For this review, take the finished solid that the model builds, in its own axes (mm). Face numbers are marked on the shaded views. A direction names the side the tool comes from. Round coordinates to 2 decimals unless told otherwise and drop trailing zeros. Write each loop counter-clockwise with the first axis right and the second up, starting at its lowest first coordinate (ties: lowest second). Pieces come first, ordered by that corner, then holes. Notation, with made-up numbers: M -20.75,-40 L -5.75,-40 A21 ccw -5.75,-4 Z; hole C 54,27 d7. An arc over 180 degrees is marked long. Use one line per item in the form item = value. Start each with the question number.
Item 1: Draft analysis for pull direction Y (two halves, no side actions). For the marked faces 6, 7, 8 and 9, state which applies: released by +Y, released by -Y, zero draft, split by the parting line, or undercut.
Item 2: Add section C-C (y = -3694). State the section outline as (x, z) points.
Item 3: For P1, Ø5, axis at x = 7373, y = -3677.5, coming from the +Z side; P2, Ø3.5, axis at x = 7512, z = 29, coming from the -Y side; P3, Ø24, axis at x = 7526.5, y = -3762, coming from the +Z side; P4, Ø3.5, axis at x = 7403.5, z = 28, coming from the -Y side, all flat-tipped, find the tip position at first contact; note any pin that passes through.
Item 4: For line 1 (Y direction, x = 7536.5, z = 31); line 2 (X direction, y = -3691, z = 32.5); line 3 (Y direction, x = 7405, z = 28), list the stretches that pass through material, from the lowest coordinate up. Write a range as [from, to].
Item 5: Add section A-A (z = 97.5). State the section outline as (x, y) points, and give its area (3 significant figures).
Item 6: For the marked faces 1, 2, 3, 4 and 5, list the 3-axis set-ups (+Z, -Z, +X, -X, +Y, -Y) from which the entire face can be reached by the end or side of a thin tool; tool diameter is ignored.
Item 7: Add section B-B (x = 7409). State the section outline as (y, z) points, and give its area (3 significant figures).
Item 8: Add section D-D (z = 14). State the section outline as (x, y) points, and give its area (3 significant figures).
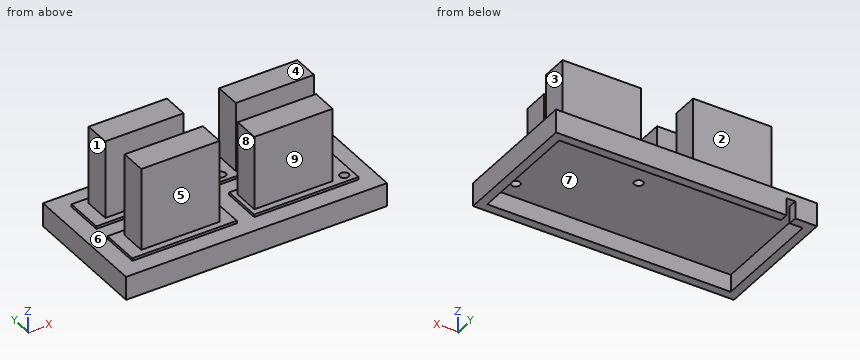
Autodesk Inventor part; units mm, degrees
ref_plane "YZ Plane" through (0, 0, 0) normal (1, 0, 0) x (0, 1, 0)
ref_plane "XZ Plane" through (0, 0, 0) normal (0, 1, 0) x (-1, 0, 0)
ref_plane "XY Plane" through (0, 0, 0) normal (0, 0, 1) x (1, 0, 0)
sketch "Skizze1" plane through (0, 0, 0) normal (0, 0, 1) x (1, 0, 0)
  line L0 (7309.0058, -3653.1811) -> (7609.0058, -3653.1811)
  line L1 (7609.0058, -3653.1811) -> (7609.0058, -3803.1811)
  line L2 (7609.0058, -3803.1811) -> (7309.0058, -3803.1811)
  line L3 (7309.0058, -3803.1811) -> (7309.0058, -3653.1811)
  point P0 (0, 0)
  dimension "d0" = 300
  dimension "d1" = 150
extrude "Extrusion1" add sketch "Skizze1" along normal blind 30
sketch "Skizze2" plane through (0, 0, 30) normal (0, 0, 1) x (1, 0, 0)
  line L0 (7309.0058, -3653.1811) -> (7309.0058, -3803.1811)
  line L1 (7609.0058, -3803.1811) -> (7609.0058, -3653.1811)
  line L2 (7309.0058, -3718.1811) -> (7609.0058, -3718.1811)
  line L3 (7609.0058, -3718.1811) -> (7609.0058, -3738.1811)
  line L4 (7609.0058, -3738.1811) -> (7309.0058, -3738.1811)
  line L5 (7309.0058, -3738.1811) -> (7309.0058, -3718.1811)
  line L6 (7609.0058, -3653.1811) -> (7309.0058, -3653.1811)
  point P0 (0, 0)
  dimension "d4" = 20
  dimension "d5" = 65
extrude "Extrusion2" cut sketch "Skizze2" against normal blind 3 contours L2 L1 L4 L0
sketch "Skizze3" plane through (0, 0, 30) normal (0, 0, 1) x (1, 0, 0)
  line L0 (7609.0058, -3653.1811) -> (7309.0058, -3653.1811)
  line L1 (7309.0058, -3803.1811) -> (7609.0058, -3803.1811)
  line L2 (7449.0058, -3653.1811) -> (7469.0058, -3653.1811)
  line L3 (7469.0058, -3653.1811) -> (7469.0058, -3803.1811)
  line L4 (7469.0058, -3803.1811) -> (7449.0058, -3803.1811)
  line L5 (7449.0058, -3803.1811) -> (7449.0058, -3653.1811)
  line L6 (7309.0058, -3653.1811) -> (7309.0058, -3718.1811)
  point P0 (0, 0)
  dimension "d8" = 20
  dimension "d9" = 140
extrude "Extrusion3" cut sketch "Skizze3" against normal blind 3
sketch "Skizze4" plane through (0, 0, 30) normal (0, 0, 1) x (1, 0, 0)
  line L0 (7609.0058, -3653.1811) -> (7309.0058, -3653.1811)
  line L1 (7309.0058, -3803.1811) -> (7609.0058, -3803.1811)
  line L2 (7609.0058, -3653.1811) -> (7589.0058, -3653.1811)
  line L3 (7589.0058, -3653.1811) -> (7589.0058, -3803.1811)
  line L4 (7589.0058, -3803.1811) -> (7609.0058, -3803.1811)
  line L5 (7609.0058, -3803.1811) -> (7609.0058, -3653.1811)
  line L6 (7309.0058, -3653.1811) -> (7329.0058, -3653.1811)
  line L7 (7329.0058, -3653.1811) -> (7329.0058, -3803.1811)
  line L8 (7329.0058, -3803.1811) -> (7309.0058, -3803.1811)
  line L9 (7309.0058, -3803.1811) -> (7309.0058, -3653.1811)
  line L10 (7309.0058, -3803.1811) -> (7609.0058, -3803.1811)
  line L11 (7609.0058, -3803.1811) -> (7609.0058, -3783.1811)
  line L12 (7609.0058, -3783.1811) -> (7309.0058, -3783.1811)
  line L13 (7309.0058, -3783.1811) -> (7309.0058, -3803.1811)
  line L14 (7609.0058, -3653.1811) -> (7309.0058, -3653.1811)
  line L15 (7309.0058, -3653.1811) -> (7309.0058, -3673.1811)
  line L16 (7309.0058, -3673.1811) -> (7609.0058, -3673.1811)
  line L17 (7609.0058, -3673.1811) -> (7609.0058, -3653.1811)
  point P0 (0, 0)
  point P1 (7589.0058, -3783.1811)
  point P2 (7329.0058, -3783.1811)
  point P3 (7329.0058, -3673.1811)
  point P4 (7589.0058, -3673.1811)
  dimension "d12" = 20
  dimension "d13" = 20
  dimension "d14" = 20
  dimension "d15" = 20
extrude "Extrusion4" cut sketch "Skizze4" against normal blind 3 contours L5 L16 L3 L0 | L3 L16 L7 L0 | L5 L12 L3 L16 | L7 L16 L9 L0 | L5 L1 L3 L12 | L7 L12 L9 L16 | L3 L1 L7 L12 | L7 L1 L9 L12
sketch "Skizze5" plane through (0, 0, 30) normal (0, 0, 1) x (1, 0, 0)
  line L0 (7344.0058, -3680.6811) -> (7434.0058, -3680.6811)
  line L1 (7434.0058, -3680.6811) -> (7434.0058, -3710.6811)
  line L2 (7434.0058, -3710.6811) -> (7344.0058, -3710.6811)
  line L3 (7344.0058, -3710.6811) -> (7344.0058, -3680.6811)
  line L4 (7449.0058, -3673.1811) -> (7329.0058, -3673.1811)
  line L5 (7329.0058, -3673.1811) -> (7329.0058, -3718.1811)
  line L6 (7344.0058, -3745.6811) -> (7434.0058, -3745.6811)
  line L7 (7434.0058, -3745.6811) -> (7434.0058, -3775.6811)
  line L8 (7434.0058, -3775.6811) -> (7344.0058, -3775.6811)
  line L9 (7344.0058, -3775.6811) -> (7344.0058, -3745.6811)
  line L10 (7449.0058, -3738.1811) -> (7329.0058, -3738.1811)
  line L11 (7449.0058, -3783.1811) -> (7449.0058, -3738.1811)
  line L12 (7474.0058, -3745.6811) -> (7564.0058, -3745.6811)
  line L13 (7564.0058, -3745.6811) -> (7564.0058, -3775.6811)
  line L14 (7564.0058, -3775.6811) -> (7474.0058, -3775.6811)
  line L15 (7474.0058, -3775.6811) -> (7474.0058, -3745.6811)
  line L16 (7589.0058, -3738.1811) -> (7469.0058, -3738.1811)
  line L17 (7469.0058, -3738.1811) -> (7469.0058, -3783.1811)
  line L18 (7494.0058, -3680.6811) -> (7584.0058, -3680.6811)
  line L19 (7584.0058, -3680.6811) -> (7584.0058, -3710.6811)
  line L20 (7584.0058, -3710.6811) -> (7494.0058, -3710.6811)
  line L21 (7494.0058, -3710.6811) -> (7494.0058, -3680.6811)
  line L22 (7589.0058, -3673.1811) -> (7469.0058, -3673.1811)
  line L23 (7589.0058, -3718.1811) -> (7589.0058, -3673.1811)
  line L24 (7609.0058, -3803.1811) -> (7309.0058, -3803.1811)
  line L25 (7309.0058, -3803.1811) -> (7309.0058, -3653.1811)
  line L26 (7609.0058, -3653.1811) -> (7609.0058, -3803.1811)
  line L27 (7309.0058, -3653.1811) -> (7609.0058, -3653.1811)
  point P0 (0, 0)
  point P1 (7329.0058, -3695.6811)
  point P2 (7564.0058, -3760.6811)
  dimension "d18" = 90
  dimension "d19" = 30
  dimension "d20" = 7.5
  dimension "d21" = 15
  dimension "d22" = 90
  dimension "d23" = 30
  dimension "d24" = 7.5
  dimension "d25" = 15
  dimension "d26" = 90
  dimension "d27" = 30
  dimension "d28" = 7.5
  dimension "d29" = 5
  dimension "d30" = 90
  dimension "d31" = 30
  dimension "d32" = 7.5
  dimension "d33" = 5
  dimension "d58" = 27.5
  dimension "d59" = 35
  dimension "d60" = 35
  dimension "d61" = 45
  dimension "d62" = 27.5
  dimension "d63" = 25
  dimension "d64" = 27.5
extrude "Extrusion5" add sketch "Skizze5" along normal blind 90 contours L0 L1 L2 L3
extrude "Extrusion6" add sketch "Skizze5" along normal blind 80 contours L18 L19 L20 L21
extrude "Extrusion7" add sketch "Skizze5" along normal blind 95 contours L6 L7 L8 L9
extrude "Extrusion8" add sketch "Skizze5" along normal blind 85 contours L12 L13 L14 L15
sketch "Skizze6" plane through (0, 0, 0) normal (0, 0, -1) x (-1, 0, 0)
  line L0 (-7599.0058, -3663.1811) -> (-7319.0058, -3663.1811)
  line L1 (-7319.0058, -3663.1811) -> (-7319.0058, -3793.1811)
  line L2 (-7319.0058, -3793.1811) -> (-7599.0058, -3793.1811)
  line L3 (-7599.0058, -3793.1811) -> (-7599.0058, -3663.1811)
  line L4 (-7609.0058, -3653.1811) -> (-7309.0058, -3653.1811)
  line L5 (-7609.0058, -3803.1811) -> (-7609.0058, -3653.1811)
  line L6 (-7344.0058, -3653.1811) -> (-7334.0058, -3653.1811)
  line L7 (-7334.0058, -3653.1811) -> (-7334.0058, -3663.1811)
  line L8 (-7334.0058, -3663.1811) -> (-7344.0058, -3663.1811)
  line L9 (-7344.0058, -3663.1811) -> (-7344.0058, -3653.1811)
  line L10 (-7309.0058, -3653.1811) -> (-7309.0058, -3803.1811)
  point P0 (0, 0)
  point P1 (-7334.0058, -3658.1811)
  dimension "d42" = 280
  dimension "d43" = 130
  dimension "d44" = 10
  dimension "d45" = 10
  dimension "d46" = 10
  dimension "d47" = 25
extrude "Extrusion9" cut sketch "Skizze6" against normal blind 20
sketch "Skizze7" plane through (0, 0, 30) normal (0, 0, 1) x (1, 0, 0)
  circle A0 centre (7479.0058, -3708.1811) radius 5
  circle A1 centre (7579.0058, -3773.1811) radius 5
  line L0 (7469.0058, -3673.1811) -> (7469.0058, -3718.1811)
  line L1 (7469.0058, -3718.1811) -> (7589.0058, -3718.1811)
  line L2 (7589.0058, -3783.1811) -> (7589.0058, -3738.1811)
  line L3 (7469.0058, -3783.1811) -> (7589.0058, -3783.1811)
  point P0 (0, 0)
  dimension "d50" = 10
  dimension "d51" = 10
  dimension "d52" = 10
  dimension "d53" = 10
  dimension "d54" = 10
  dimension "d55" = 10
extrude "Extrusion10" cut sketch "Skizze7" against normal through all
sketch "Skizze8" plane through (0, 0, 20) normal (0, 0, -1) x (-1, 0, 0)
  line L0 (-7349.0058, -3685.6811) -> (-7429.0058, -3685.6811)
  line L1 (-7429.0058, -3685.6811) -> (-7429.0058, -3705.6811)
  line L2 (-7429.0058, -3705.6811) -> (-7349.0058, -3705.6811)
  line L3 (-7349.0058, -3705.6811) -> (-7349.0058, -3685.6811)
  line L4 (-7609.0058, -3653.1811) -> (-7344.0058, -3653.1811)
  line L5 (-7309.0058, -3653.1811) -> (-7309.0058, -3803.1811)
  line L6 (-7349.0058, -3770.6811) -> (-7429.0058, -3770.6811)
  line L7 (-7429.0058, -3770.6811) -> (-7429.0058, -3750.6811)
  line L8 (-7429.0058, -3750.6811) -> (-7349.0058, -3750.6811)
  line L9 (-7349.0058, -3750.6811) -> (-7349.0058, -3770.6811)
  line L10 (-7309.0058, -3803.1811) -> (-7609.0058, -3803.1811)
  line L11 (-7559.0058, -3770.6811) -> (-7479.0058, -3770.6811)
  line L12 (-7479.0058, -3770.6811) -> (-7479.0058, -3750.6811)
  line L13 (-7479.0058, -3750.6811) -> (-7559.0058, -3750.6811)
  line L14 (-7559.0058, -3750.6811) -> (-7559.0058, -3770.6811)
  line L15 (-7609.0058, -3803.1811) -> (-7609.0058, -3653.1811)
  line L16 (-7499.0058, -3705.6811) -> (-7579.0058, -3705.6811)
  line L17 (-7579.0058, -3705.6811) -> (-7579.0058, -3685.6811)
  line L18 (-7579.0058, -3685.6811) -> (-7499.0058, -3685.6811)
  line L19 (-7499.0058, -3685.6811) -> (-7499.0058, -3705.6811)
  point P0 (0, 0)
  dimension "d65" = 80
  dimension "d66" = 20
  dimension "d67" = 32.5
  dimension "d68" = 40
  dimension "d69" = 80
  dimension "d70" = 20
  dimension "d71" = 40
  dimension "d72" = 32.5
  dimension "d73" = 80
  dimension "d74" = 50
  dimension "d75" = 32.5
  dimension "d76" = 80
  dimension "d77" = 20
  dimension "d78" = 32.5
  dimension "d79" = 30
extrude "Extrusion11" add sketch "Skizze8" against normal blind 70
properties part number "2"
Calculated:
q1.face_6 = undercut
q1.face_7 = undercut
q1.face_8 = zero draft
q1.face_9 = released by -Y
q2.outline = M 7309.01,0 L 7319.01,0 L 7319.01,20 L 7599.01,20 L 7599.01,0 L 7609.01,0 L 7609.01,27 L 7589.01,27 L 7589.01,30 L 7584.01,30 L 7584.01,110 L 7494.01,110 L 7494.01,30 L 7469.01,30 L 7469.01,27 L 7449.01,27 L 7449.01,30 L 7434.01,30 L 7434.01,120 L 7344.01,120 L 7344.01,30 L 7329.01,30 L 7329.01,27 L 7309.01,27 Z
q3.P1 = 30
q3.P2 = -3783.18
q3.P3 = 115
q3.P4 = -3803.18
q4.line_1 = [-3775.68, -3745.68], [-3710.68, -3680.68]
q4.line_2 = [7344.01, 7434.01], [7494.01, 7584.01]
q4.line_3 = [-3783.18, -3738.18], [-3718.18, -3673.18]
q5.outline = M 7344.01,-3775.68 L 7434.01,-3775.68 L 7434.01,-3745.68 L 7344.01,-3745.68 Z; M 7344.01,-3710.68 L 7434.01,-3710.68 L 7434.01,-3680.68 L 7344.01,-3680.68 Z; M 7474.01,-3775.68 L 7564.01,-3775.68 L 7564.01,-3745.68 L 7474.01,-3745.68 Z; M 7494.01,-3710.68 L 7584.01,-3710.68 L 7584.01,-3680.68 L 7494.01,-3680.68 Z
q5.area = 10,800 mm^2
q6.face_1 = +Z, -X, +Y, -Y
q6.face_2 = +Z, +X, -X, +Y
q6.face_3 = +Z, +X, +Y, -Y
q6.face_4 = +Z, +X, +Y
q6.face_5 = +Z, +X, -X, -Y
q7.outline = M -3803.18,0 L -3793.18,0 L -3793.18,20 L -3663.18,20 L -3663.18,0 L -3653.18,0 L -3653.18,27 L -3673.18,27 L -3673.18,30 L -3680.68,30 L -3680.68,120 L -3710.68,120 L -3710.68,30 L -3718.18,30 L -3718.18,27 L -3738.18,27 L -3738.18,30 L -3745.68,30 L -3745.68,125 L -3775.68,125 L -3775.68,30 L -3783.18,30 L -3783.18,27 L -3803.18,27 Z
q7.area = 7,270 mm^2
q8.outline = M 7309.01,-3803.18 L 7609.01,-3803.18 L 7609.01,-3653.18 L 7344.01,-3653.18 L 7344.01,-3663.18 L 7599.01,-3663.18 L 7599.01,-3793.18 L 7319.01,-3793.18 L 7319.01,-3663.18 L 7334.01,-3663.18 L 7334.01,-3653.18 L 7309.01,-3653.18 Z
q8.area = 8,500 mm^2
